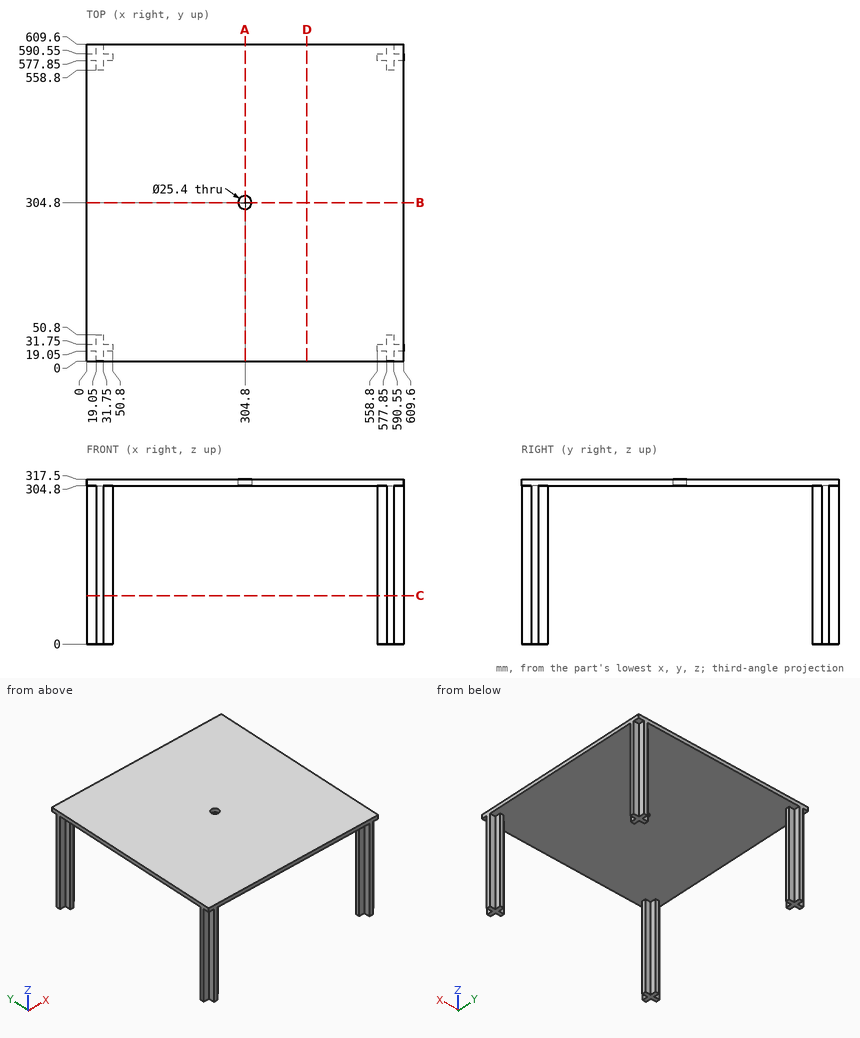
Print and shaded views of the part. All mm, measured from the part's lowest x, y and z. Round coordinates to 2 decimals unless told otherwise and drop trailing zeros. Write each loop counter-clockwise with the first axis right and the second up, starting at its lowest first coordinate (ties: lowest second). Pieces come first, ordered by that corner, then holes. Notation, with made-up numbers: M 21.25,9 L 43.25,9 A21 cw 43.25,41 Z; hole C -23,65 d11. An arc over 180 degrees is marked long. Use a Markdown table: item, result. Add a question column.
1. Flat gauge pins, fed straight in: P1, Ø4, axis at y = 27, z = 160, coming from the -X side; P2, Ø2, axis at x = 143.5, y = 264, coming from the -Z side; P3, Ø5.5, axis at y = 600, z = 98.5, coming from the +X side; P4, Ø5.5, axis at x = 572, z = 109.5, coming from the +Y side. Where does each tip first touch, or does it go through?
2. Slice it at A-A on x = 304.8. Give the cut face in (y, z).
3. Slice it at D-D on x = 424. Give the cut face in (y, z), then the cut area to 3 significant figures.
4. Drill centre lines: probe 1 along Y at (x, z) = (304, 308); probe 2 along Z at (x, y) = (441, 511.5). Where is each one in solid material? Low to high.
5. Slice it at C-C on z = 93. Give the number of separate pieces and of enclosed holes in the cut face, then the cut area to 3 significant figures.
Reply:
| question | item | result |
|---|---|---|
| 1 | P1 | stops at x = 0 |
| 1 | P2 | stops at z = 304.8 |
| 1 | P3 | stops at x = 590.55 |
| 1 | P4 | stops at y = 590.55 |
| 2 | outline | M 0,304.8 L 292.1,304.8 L 292.1,317.5 L 0,317.5 Z; M 317.5,304.8 L 609.6,304.8 L 609.6,317.5 L 317.5,317.5 Z |
| 3 | outline | M 0,304.8 L 609.6,304.8 L 609.6,317.5 L 0,317.5 Z |
| 3 | area | 7,740 mm^2 |
| 4 | probe 1 | y = 0 to 292.13, 317.47 to 609.6 |
| 4 | probe 2 | z = 304.8 to 317.5 |
| 5 | separate pieces | 4 |
| 5 | enclosed holes | 0 |
| 5 | area | 4,520 mm^2 |
